```python
from build123d import *

# Parameters (mm, degrees)
SKETCH1_W           = 210
SKETCH1_H           = 120
BOSS_EXTRUDE1_DEPTH = 50
SKETCH2_W           = 105
SKETCH2_H           = 120
BOSS_EXTRUDE2_DEPTH = 18
SKETCH3_R           = 20
BOSS_EXTRUDE3_DEPTH = 10
SKETCH4_R           = 20
BOSS_EXTRUDE4_DEPTH = 10


with BuildPart() as part:
    # Sketch1 → Boss-Extrude1 (new body)
    with BuildSketch(Plane(origin=(0, 0, 0), x_dir=(1, 0, 0), z_dir=(0, 1, 0))):
        Rectangle(SKETCH1_W, SKETCH1_H)
    extrude(amount=BOSS_EXTRUDE1_DEPTH)

    # Sketch2 → Boss-Extrude2 (add)
    with BuildSketch(Plane(origin=(0, 50, 0), x_dir=(1, 0, 0), z_dir=(0, 1, 0))):
        with Locations((-52.5, 0)):
            Rectangle(SKETCH2_W, SKETCH2_H)
    extrude(amount=BOSS_EXTRUDE2_DEPTH)

    # Sketch3 → Boss-Extrude3 (add)
    with BuildSketch(Plane(origin=(0, 68, 0), x_dir=(1, 0, 0), z_dir=(0, 1, 0))):
        with Locations(Location((-51, 0, 0), (0, 0, 270))):
            Circle(SKETCH3_R)
    extrude(amount=BOSS_EXTRUDE3_DEPTH)

    # Sketch4 → Boss-Extrude4 (add)
    with BuildSketch(Plane(origin=(0, 50, 0), x_dir=(1, 0, 0), z_dir=(0, 1, 0))):
        with Locations(Location((51, 0, 0), (0, 0, 270))):
            Circle(SKETCH4_R)
    extrude(amount=BOSS_EXTRUDE4_DEPTH)


solid = part.part
```
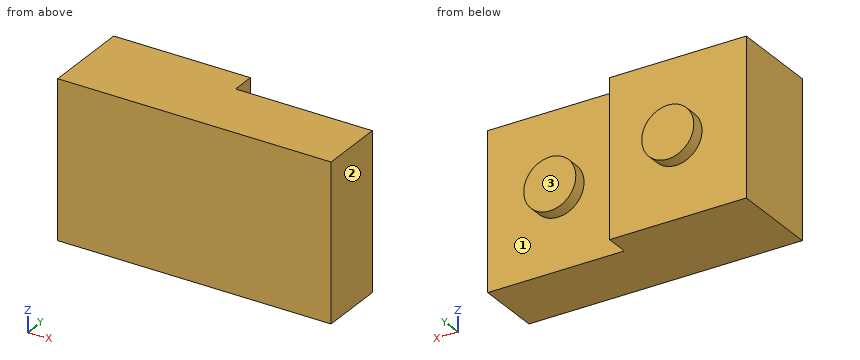
Geometry check sheet. Reference: the model listing, model coordinates, mm. Face numbers are marked on the shaded views. A direction names the side the tool comes from. Coordinates: 2 decimals unless noted, no trailing zeros. Loops run counter-clockwise (first coordinate to the right, second up) from the corner with the lowest first, then second, coordinate; pieces in that order, holes last.
Item 1: Thickness scan on line 1 (Y direction, x = 70.5, z = -28.5); line 2 (Y direction, x = -86.5, z = -1.5); line 3 (X direction, y = 57, z = -34.5). Record the ranges inside material, lowest first.
Item 2: Access from +Z, -Z, +X, -X, +Y, -Y to the whole of each face (thin tool, end or side, straight path). Record for the marked faces 1, 2 and 3.
Item 3: Sectioned sample at D-D, the plane z = 31. Record the boundary of the cut face in (x, y), then the cut area to 3 significant figures.
Item 4: Go/stop test with flat-tipped pins: pin 1 Ø1.5 at (x, z) = (-63.5, 15) entering from -Y; pin 2 Ø2 at (x, z) = (29.5, 28.5) entering from +Y; pin 3 Ø20 at (x, z) = (54.5, 2.5) entering from +Y. Record where each tip stops, or that it passes through.
Item 5: Sectioned sample at B-B, the plane x = -51. Record the boundary of the cut face in (y, z).
Item 6: Sectioned sample at C-C, the plane x = 40. Record the boundary of the cut face in (y, z), then the cut area to 3 significant figures.
Item 7: Sectioned sample at A-A, the plane z = 0. Record the boundary of the cut face in (x, y).
Check result:
1. line 1: y = 0 to 50
1. line 2: y = 0 to 68
1. line 3: x = -105 to 0
2. face 1: +Y
2. face 2: +Z, -Z, +X, +Y, -Y
2. face 3: +Z, -Z, +X, +Y
3. outline: (-105, 0) - (105, 0) - (105, 50) - (0, 50) - (0, 68) - (-105, 68) - close
3. area: 12,400 mm2
4. pin 1: stops at y = 0
4. pin 2: stops at y = 50
4. pin 3: stops at y = 60
5. outline: (0, -60) - (68, -60) - (68, -20) - (78, -20) - (78, 20) - (68, 20) - (68, 60) - (0, 60) - close
6. outline: (0, -60) - (50, -60) - (50, -16.7) - (60, -16.7) - (60, 16.7) - (50, 16.7) - (50, 60) - (0, 60) - close
6. area: 6,330 mm2
7. outline: (-105, 0) - (105, 0) - (105, 50) - (71, 50) - (71, 60) - (31, 60) - (31, 50) - (0, 50) - (0, 68) - (-31, 68) - (-31, 78) - (-71, 78) - (-71, 68) - (-105, 68) - close
